```python
from build123d import *

# Parameters (mm, degrees)
F0_W     = 50.8
F0_H     = 50.8
F1_DEPTH = 3.175
F2_W     = 57.15
F2_H     = 88.9
F3_DEPTH = 3.175
F4_W     = 57.15
F4_H     = 88.9
F5_DEPTH = 3.175
F6_W     = 50.8
F6_H     = 88.9
F7_DEPTH = 3.175
F8_W     = 50.8
F8_H     = 88.9
F9_DEPTH = 3.175


with BuildPart() as f1:
    # F0 (on Top) → F1 (new body)
    with BuildSketch(Plane.XY):
        Rectangle(F0_W, F0_H)
    extrude(amount=F1_DEPTH)

    # F2 (on face) → F3 (join)
    with BuildSketch(Plane.XZ.offset(25.4)):
        with Locations((0, 44.45)):
            Rectangle(F2_W, F2_H)
    extrude(amount=F3_DEPTH)

    # F4 (on face) → F5 (join)
    with BuildSketch(Plane(origin=(0, 25.4, 0), x_dir=(-1, 0, 0), z_dir=(0, 1, 0))):
        with Locations((0, 44.45)):
            Rectangle(F4_W, F4_H)
    extrude(amount=F5_DEPTH)

    # F6 (on face) → F7 (join)
    with BuildSketch(Plane(origin=(-25.4, 0, 0), x_dir=(0, -1, 0), z_dir=(-1, 0, 0))):
        with Locations((0, 44.45)):
            Rectangle(F6_W, F6_H)
    extrude(amount=F7_DEPTH)

    # F8 (on face) → F9 (join)
    with BuildSketch(Plane.YZ.offset(25.4)):
        with Locations((0, 44.45)):
            Rectangle(F8_W, F8_H)
    extrude(amount=F9_DEPTH)


solid = f1.part
```
Design review of the part built by this model. Coordinates are the model's own, in mm. A direction names the side the tool comes from. Give positions to 0.01 mm unless a question says otherwise; leave off trailing zeros. Order: outer loops, then holes, each group sorted by start corner. A loop starts at its lowest first (then second) coordinate and runs counter-clockwise, first axis right, second up. Notation, with made-up numbers: (83, 2) - (100, 2) arc R29 ccw to (100, 22) - close; hole circle Ø8 at (1, -39.5). An arc over 180 degrees is marked (long way). Use a Markdown table: item, result. Add a question column.
(1) Mouldability with a two-part tool opening along X and no side actions: class faces 1 (the face through (-25.4, 0, 47)), 2 (the face through (-4, -26, 88.9)), 3 (the face through (28.575, 0, 45)), 4 (the face through (0, 25.4, 47)) as +X half, -X half, draft (parallel to the pull), parting line (faces both ways), or undercut.
(2) Clearance check with flat-ended pins moving along their axes: P1, Ø4, axis at x = -10.5, y = 12.5, coming from the -Z side; P2, Ø5, axis at x = -4.5, y = 5, coming from the +Z side (3 decimals). State where each tip first meets the part, or that it passes through.
(3) Add section A-A on x = 11.5. Give the boundary of the cut face in (y, z) (3 decimals).
(4) Machinability: for faces 5 (the face through (0, -25.4, 47)), 6 (the face through (-28.575, 0, 45)), which of the approach directions +Z, -Z, +X, -X, +Y, -Y give a long, thin tool a straight path to every point of the face, cutting with its end or side? Answer none if there is none.
(5) Add section B-B on z = 11. Give the boundary of the cut face in (x, y) (3 decimals), then the cut area to 3 significant figures.
(6) Wall thickness on probe 1 along X at (y, z) = (-13.5, 20.5) (3 decimals); probe 2 along Z at (x, y) = (-11, 3.5) (3 decimals): over which ranges is each line inside the solid? List them lowest first. Write a range as [from, to].
Report:
| question | item | result |
|---|---|---|
| 1 | face 1 | undercut |
| 1 | face 2 | draft |
| 1 | face 3 | +X half |
| 1 | face 4 | undercut |
| 2 | P1 | stops at z = 0 |
| 2 | P2 | stops at z = 3.175 |
| 3 | outline | (-28.575, 0) - (28.575, 0) - (28.575, 88.9) - (25.4, 88.9) - (25.4, 3.175) - (-25.4, 3.175) - (-25.4, 88.9) - (-28.575, 88.9) - close |
| 4 | face 5 | +Z |
| 4 | face 6 | +Z, -Z, -X, +Y, -Y |
| 5 | outline | (-28.575, -28.575) - (28.575, -28.575) - (28.575, 28.575) - (-28.575, 28.575) - close; hole (-25.4, -25.4) - (25.4, -25.4) - (25.4, 25.4) - (-25.4, 25.4) - close |
| 5 | area | 685 mm² |
| 6 | probe 1 | x = [-28.575, -25.4], [25.4, 28.575] |
| 6 | probe 2 | z = [0, 3.175] |
